CAD build for the part. Positions are in the model's coordinates, mm. Face numbers are marked on the shaded views. A direction names the side the tool comes from. Round coordinates to 2 decimals unless told otherwise and drop trailing zeros. Loops run counter-clockwise (first coordinate to the right, second up) from the corner with the lowest first, then second, coordinate; pieces in that order, holes last. Notation, with made-up numbers: M 86.5,-36.75 L 123.5,-36.75 A23 cw 123.5,0.25 Z; hole C 32.5,-10.5 d8. An arc over 180 degrees is marked long. Use one line per item in the form item = value.
from build123d import *

# Parameters (mm, degrees)
F1_DEPTH = 180


with BuildPart() as f1:
    # F0 (on Top) → F1 (new body)
    with BuildSketch(Plane.XY):
        with BuildLine():
            Line((53.880711, -50), (63.297123, -50))
            Line((63.297123, -50), (63.297123, 0))
            Line((63.297123, 0), (63.297123, 2.555883))
            ThreePointArc((63.297123, 2.555883), (54.874784, 30.426908), (33.319647, 50))
            Line((33.319647, 50), (-33.05907, 50))
            ThreePointArc((-33.05907, 50), (-53.687577, 28.331919), (-63.297123, 0))
            Line((-63.297123, 0), (-63.297123, -50))
            Line((-63.297123, -50), (-53.297123, -50))
            Line((-53.297123, -50), (-53.297123, 0))
            ThreePointArc((-53.297123, 0), (-47.239503, 22.95935), (-30.643604, 39.941771))
            Line((-30.643604, 39.941771), (35.021361, 39.941771))
            ThreePointArc((35.021361, 39.941771), (48.928843, 22.085177), (53.880711, 0))
            Line((53.880711, 0), (53.880711, -50))
        make_face()
    extrude(amount=F1_DEPTH)


solid = f1.part
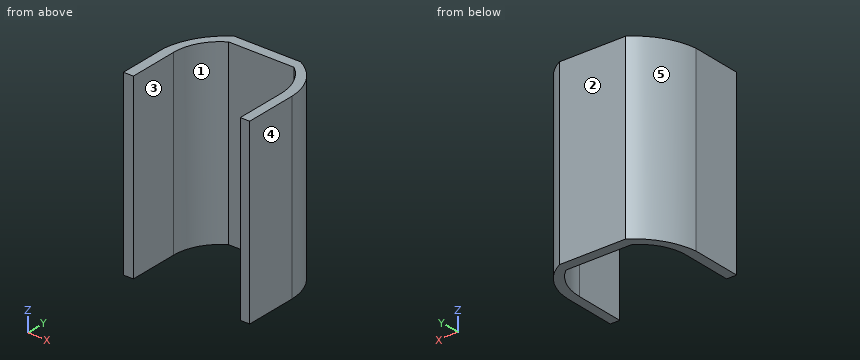
1. Pull direction X, two halves, no side cores. Call the marked faces 3, 4 and 5: +X half, -X half, draft (parallel to the pull), parting line (faces both ways), or undercut.
Completed:
face_3 = undercut
face_4 = +X half
face_5 = -X half
2. Probe line 1 along X through (y, z) = (-4.5, 8.5); line 2 along Y through (x, z) = (-16, 119); line 3 along X through (y, z) = (4.5, 100). List the from-to ranges inside material, lowest first. Write a range as from..to.
Completed:
line_1 = -63.3..-53.3, 53.88..63.3
line_2 = 39.94..50
line_3 = -62.65..-53.08, 53.68..63.22
3. Cut at C-C on y = 9. Write the cut outline in (x, z).
Completed:
outline = M -61.7,0 L -52.42,0 L -52.42,180 L -61.7,180 Z; M 53.09,0 L 62.76,0 L 62.76,180 L 53.09,180 Z
4. Cut at D-D on x = 16. Write the cut outline in (y, z).
Completed:
outline = M 39.94,0 L 50,0 L 50,180 L 39.94,180 Z
5. Tool access for the marked faces 1 and 2: list every direction of +Z, -Z, +X, -X, +Y, -Y with a clear straight run to the whole face (end or side of a thin tool).
Completed:
face_1 = +Z, -Z, -Y
face_2 = +Z, -Z, +X, -X, +Y
6. Cut at A-A on y = -35.5. Write the cut outline in (x, z), and give its area (3 significant figures).
Completed:
outline = M -63.3,0 L -53.3,0 L -53.3,180 L -63.3,180 Z; M 53.88,0 L 63.3,0 L 63.3,180 L 53.88,180 Z
area = 3,490 mm2
7. Cut at B-B on z = 78.5. Write the cut outline in (x, y).
Completed:
outline = M -63.3,-50 L -53.3,-50 L -53.3,0 A46.54 cw -30.64,39.94 L 35.02,39.94 A51.73 cw 53.88,0 L 53.88,-50 L 63.3,-50 L 63.3,2.56 A54.57 ccw 33.32,50 L -33.06,50 A69.51 ccw -63.3,0 Z
8. Drop a flat-ended pin along its axis: P1, Ø8, axis at x = 14.5, z = 84, coming from the -Y side. Give the stop position or say it passes through.
Completed:
P1 = 39.94
